The listing builds one solid part. Answer for the finished solid, in the listing's coordinates (mm). Round coordinates to 2 decimals unless told otherwise and drop trailing zeros. Order: outer loops, then holes, each group sorted by start corner. A loop starts at its lowest first (then second) coordinate and runs counter-clockwise, first axis right, second up. Notation, with made-up numbers: (0, -34) - (51, -34) arc R15 ccw to (51, -30) - close; hole circle Ø5 at (-0.75, 23). An arc over 180 degrees is marked (long way). Use CSV: the item, a comma, the result in double quotes. Start each with the question number.
Item 1: Find section A-A, the plane x = 0. Give the vertices of the cut face in (y, z).
Item 2: Straight lines are drawn through the part: line 1 along Z through (x, y) = (0, -2); line 2 along Z through (x, y) = (13.5, -22); line 3 along X through (y, z) = (4, 20.5). For each, find the intervals that lie inside material, in ascending order. Write a range as [from, to].
Item 3: Flat-ended cylindrical pins translate along their axes: P1, Ø4, axis at x = -11.5, z = 39.5, coming from the +Y side; P2, Ø5, axis at x = -18, z = 32, coming from the +Y side. Find the tip coordinate at first contact, or state that the pin passes through.
Item 4: Determine the mould class of faces 1 (the flat face through (-30, 0, 30)), 2 (the flat face through (0, 23, 3)), 3 (the cylindrical face through (7.48, -0.28, 18.77)), 4 (the flat face through (-27, 0, 58)) for opening direction Z: +Z half, -Z half, draft (parallel to the pull), parting line (faces both ways), or undercut.
Item 5: Find section B-B, the plane y = -5. Give the vertices of the cut face in (x, z).
```python
from build123d import *

# Parameters (mm, degrees)
F0_W     = 60
F0_H     = 50
F1_DEPTH = 60
F2_R     = 16.203635
F3_DEPTH = 50.001
F4_R     = 5
F5_SIZE  = 5


with BuildPart() as f1:
    # F0 (on Top) → F1 (new body)
    with BuildSketch(Plane.XY):
        Rectangle(F0_W, F0_H)
    extrude(amount=F1_DEPTH)

    # F2 (on face) → F3 (cut, through all)
    with BuildSketch(Plane.XZ.offset(25)):
        with Locations((0, 33.142988)):
            Circle(F2_R)
    extrude(amount=-F3_DEPTH, mode=Mode.SUBTRACT)

    # F4
    f4_edges = [f1.edges().sort_by_distance(p)[0] for p in [
        (-16.203635, -25, 33.142988),
        (-16.203635, 25, 33.142988),
    ]]
    fillet(f4_edges, radius=F4_R)

    # F5
    f5_edges = [f1.edges().sort_by_distance(p)[0] for p in [
        (-30, 25, 30),
        (-30, -25, 30),
        (-30, 0, 60),
        (0, 25, 60),
        (0, -25, 60),
        (0, -25, 0),
        (-30, 0, 0),
        (30, -25, 30),
        (30, 0, 60),
        (30, 25, 30),
        (30, 0, 0),
        (0, 25, 0),
    ]]
    chamfer(f5_edges, length=F5_SIZE)


solid = f1.part
```
Worked out:
1,outline,"(-25, 5) - (-20, 0) - (20, 0) - (25, 5) - (25, 11.94) arc R5 ccw to (20, 16.94) - (-20, 16.94) arc R5 ccw to (-25, 11.94) - close; (-25, 54.35) arc R5 ccw to (-20, 49.35) - (20, 49.35) arc R5 ccw to (25, 54.35) - (25, 55) - (20, 60) - (-20, 60) - (-25, 55) - close"
2,line 1,"z = [0, 16.94], [49.35, 60]"
2,line 2,"z = [2, 23.45], [42.84, 58]"
2,line 3,"x = [-30, -10.13], [10.13, 30]"
3,P1,"passes through"
3,P2,"stops at y = 24.96"
4,face 1,"draft"
4,face 2,"-Z half"
4,face 3,"undercut"
4,face 4,"+Z half"
5,outline,"(-30, 5) - (-25, 0) - (25, 0) - (30, 5) - (30, 55) - (25, 60) - (-25, 60) - (-30, 55) - close; hole circle Ø32.41 at (0, 33.14)"
